CAD build for the part. Positions are in the model's coordinates, mm. Face numbers are marked on the shaded views. A direction names the side the tool comes from. Round coordinates to 2 decimals unless told otherwise and drop trailing zeros. Loops run counter-clockwise (first coordinate to the right, second up) from the corner with the lowest first, then second, coordinate; pieces in that order, holes last.
from build123d import *

# Parameters (mm, degrees)
SKETCH008_W     = 125
SKETCH008_H     = 60
PAD007_DEPTH    = 15
SKETCH009_W     = 115
SKETCH009_H     = 45
POCKET001_DEPTH = 10
SKETCH010_W     = 5
SKETCH010_H     = 45
PAD008_DEPTH    = 10
PAD009_DEPTH    = 15
PAD010_DEPTH    = 25
POCKET002_DEPTH = 122.392039
POCKET003_DEPTH = 62
PAD011_DEPTH    = 25
POCKET004_DEPTH = 22
FILLET006_R     = 1
FILLET007_R     = 1
FILLET008_R     = 1
FILLET009_R     = 1
FILLET010_R     = 2
PAD012_DEPTH    = 40
SKETCH019_W     = 26.11364
SKETCH019_H     = 14.637775
POCKET005_DEPTH = 11
POCKET006_DEPTH = 12
FILLET011_R     = 2
FILLET012_R     = 2


with BuildPart() as part:
    # Sketch008 → Pad007 (new body)
    with BuildSketch(Plane.XY):
        with Locations((97.753377, 76.478924)):
            Rectangle(SKETCH008_W, SKETCH008_H)
    extrude(amount=PAD007_DEPTH)

    # Sketch009 (on Face6 of Pad007) → Pocket001 (cut)
    with BuildSketch(Plane.XY.offset(15)):
        with Locations((97.753377, 73.978924)):
            Rectangle(SKETCH009_W, SKETCH009_H)
    extrude(amount=-POCKET001_DEPTH, mode=Mode.SUBTRACT)

    # Sketch010 (on Face11 of Pocket001) → Pad008 (join)
    with BuildSketch(Plane.XY.offset(5)):
        with Locations((97.753377, 73.978924)):
            Rectangle(SKETCH010_W, SKETCH010_H)
    extrude(amount=PAD008_DEPTH)

    # Sketch011 (on Face4 of Pad008) → Pad009 (join)
    with BuildSketch(Plane(origin=(0, 0, 0), x_dir=(1, 0, 0), z_dir=(0, 0, -1))):
        Polygon((40.253377, -103.478924), (155.253377, -103.478924), (142.543141, -146.646619), (97.753377, -168.869964), (52.963613, -146.646619), align=None)
    extrude(amount=-PAD009_DEPTH)

    # Sketch012 (on Face10 of Pad009) → Pad010 (join)
    with BuildSketch(Plane(origin=(0, 0, 0), x_dir=(1, 0, 0), z_dir=(0, 0, -1))):
        Polygon((35.753377, -91.478924), (35.753377, -61.478924), (36.388107, -46.478925), (9.764659, -46.478925), (-16.208147, -61.478924), (-16.208147, -91.478924), (9.764667, -106.478923), (35.753377, -106.478923), align=None)
    extrude(amount=-PAD010_DEPTH)

    # Sketch014 (on Face12 of Pad010) → Pocket002 (cut, through all)
    with BuildSketch(Plane.XZ.offset(-46.478925)):
        Polygon((21.625628, 4), (31.014697, 39.040485), (16.014696, 39.040485), (6.625628, 34.478157), (6.625628, 4), align=None)
    extrude(amount=-POCKET002_DEPTH, mode=Mode.SUBTRACT)

    # Sketch015 (on Face8 of Pocket002) → Pocket003 (cut)
    with BuildSketch(Plane.XZ.offset(-46.478925)):
        Polygon((2.97068, 27.121502), (-3.224708, 4), (-11.224708, 4), (-11.224708, 27.121502), align=None)
    extrude(amount=-POCKET003_DEPTH, mode=Mode.SUBTRACT)

    # Sketch016 (on Face2 of Pocket003) → Pad011 (join)
    with BuildSketch(Plane(origin=(0, 0, 0), x_dir=(1, 0, 0), z_dir=(0, 0, -1))):
        with BuildLine():
            ThreePointArc((160.253377, -106.478924), (190.253377, -76.478924), (160.253377, -46.478924))
            Line((160.253377, -46.478924), (158.253377, -46.478924))
            Line((158.253377, -46.478924), (158.253377, -106.478924))
            Line((158.253377, -106.478924), (160.253377, -106.478924))
        make_face()
    extrude(amount=-PAD011_DEPTH)

    # Sketch017 (on Face34 of Pad011) → Pocket004 (cut)
    with BuildSketch(Plane.XY.offset(25)):
        with BuildLine():
            ThreePointArc((160.253377, 49.478924), (187.253377, 76.478924), (160.253377, 103.478924))
            Line((160.253377, 103.478924), (160.253377, 49.478924))
        make_face()
    extrude(amount=-POCKET004_DEPTH, mode=Mode.SUBTRACT)

    # Fillet006
    fillet006_edges = [part.edges().sort_by_distance(p)[0] for p in [
        (158.253377, 76.478924, 25),
    ]]
    fillet(fillet006_edges, radius=FILLET006_R)

    # Fillet007
    fillet007_edges = [part.edges().sort_by_distance(p)[0] for p in [
        (31.502969, 106.478923, 25),
        (27.252561, 76.478924, 25),
        (31.820334, 46.478925, 25),
        (36.070742, 53.978925, 25),
        (35.753377, 83.978924, 25),
    ]]
    fillet(fillet007_edges, radius=FILLET007_R)

    # Fillet008
    fillet008_edges = [part.edges().sort_by_distance(p)[0] for p in [
        (2.402225, 76.478922, 25),
        (4.513926, 49.511365, 25),
        (6.625628, 76.478922, 25),
        (4.513926, 103.446479, 25),
    ]]
    fillet(fillet008_edges, radius=FILLET008_R)

    # Fillet009
    fillet009_edges = [part.edges().sort_by_distance(p)[0] for p in [
        (-16.208147, 76.478924, 25),
        (-13.716428, 60.039889, 25),
        (-11.224708, 76.478924, 25),
        (-13.716428, 92.917959, 25),
    ]]
    fillet(fillet009_edges, radius=FILLET009_R)

    # Fillet010
    fillet010_edges = [part.edges().sort_by_distance(p)[0] for p in [
        (127.753377, 51.478924, 15),
        (155.253377, 73.978924, 15),
        (100.253377, 73.978924, 15),
        (95.253377, 73.978924, 15),
        (67.753377, 51.478924, 15),
        (40.253377, 73.978924, 15),
    ]]
    fillet(fillet010_edges, radius=FILLET010_R)

    # Sketch018 (on DatumPlane) → Pad012 (join)
    with BuildSketch(Plane(origin=(138.35197, 76.478924, 12.5), x_dir=(0, 0, -1), z_dir=(1, 0, 0))):
        Polygon((0, 32.455163), (-41.423717, 43.554615), (0, 43.554615), align=None)
    extrude(amount=-PAD012_DEPTH)

    # Sketch019 (on Face25 of Pad012) → Pocket005 (cut)
    with BuildSketch(Plane(origin=(0, 120.033539, 0), x_dir=(-1, 0, 0), z_dir=(0, 1, 0))):
        with Locations((-120.645542, 22.318887)):
            Rectangle(SKETCH019_W, SKETCH019_H)
    extrude(amount=-POCKET005_DEPTH, mode=Mode.SUBTRACT)

    # Sketch020 (on Face47 of Pocket005) → Pocket006 (cut)
    with BuildSketch(Plane.XY.offset(15)):
        Polygon((50.450993, 122.512529), (145.055761, 122.512529), (138.543141, 144.6313), (97.753377, 164.869964), (56.963613, 144.6313), align=None)
    extrude(amount=-POCKET006_DEPTH, mode=Mode.SUBTRACT)

    # Fillet011
    fillet011_edges = [part.edges().sort_by_distance(p)[0] for p in [
        (53.707303, 133.571915, 15),
        (77.358495, 154.750632, 15),
        (118.148259, 154.750632, 15),
        (141.799451, 133.571915, 15),
    ]]
    fillet(fillet011_edges, radius=FILLET011_R)

    # Fillet012
    fillet012_edges = [part.edges().sort_by_distance(p)[0] for p in [
        (118.35197, 120.033539, 53.923717),
    ]]
    fillet(fillet012_edges, radius=FILLET012_R)


solid = part.part
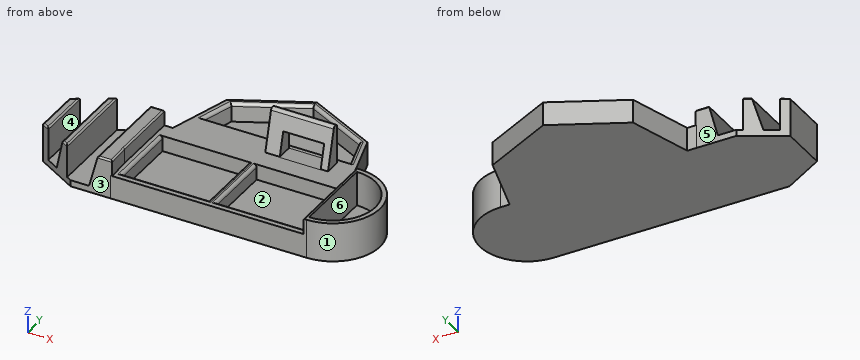
Item 1: Cut at C-C (z = 36). List the corners of the cut face in (x, y).
Verdict:
outline: (98.35, 115.23) - (138.35, 115.23) - (138.35, 120.03) - (98.35, 120.03) - close
Item 2: Flat gauge pins, fed straight in: P1, Ø4, axis at x = 72, z = 8.5, coming from the +Y side; P2, Ø4, axis at x = 75.5, y = 145.5, coming from the -Z side; P3, Ø1, axis at y = 93, z = 11.5, coming from the +X side; P4, Ø22, axis at y = 69.5, z = 17.5, coming from the +X side. Where does each tip first touch, or does it go through?
Verdict:
P1: stops at y = 157.08
P2: stops at z = 0
P3: stops at x = 185.62
P4: stops at x = 190.25
Item 3: Wall check: L1, parallel to Y at x = 120, z = 13; L2, parallel to X at y = 66.5, z = 9.5; L3, parallel to Y at x = 113, z = 7.5. Give the ranges that are in metal, low to high.
Verdict:
L1: y = 46.48 to 51.48, 96.48 to 122.51, 153.83 to 157.83
L2: x = -16.21 to -11.22, -1.75 to 6.63, 23.1 to 40.25, 95.25 to 100.25, 155.25 to 160.25, 185.34 to 188.55
L3: y = 46.48 to 51.48, 96.48 to 122.51, 157.31 to 161.31
Item 4: Cut at A-A (z = 21.5). List the corners of the cut face in (x, y).
Verdict:
outline: (-16.21, 61.48) - (-11.22, 58.6) - (-11.22, 94.36) - (-16.21, 91.48) - close; (1.46, 51.27) - (6.63, 48.29) - (6.63, 104.67) - (1.46, 101.69) - close; (26.31, 46.48) - (36.39, 46.48) - (35.75, 61.48) - (35.75, 106.48) - (26.31, 106.48) - close; (98.35, 111.35) - (107.59, 111.35) - (107.59, 120.03) - (98.35, 120.03) - close; (133.7, 111.35) - (138.35, 111.35) - (138.35, 120.03) - (133.7, 120.03) - close; (158.25, 46.48) - (160.25, 46.48) arc R30 ccw to (160.25, 106.48) - (158.25, 106.48) - close; hole (160.25, 49.48) arc R27 ccw to (160.25, 103.48) - close
Item 5: Cut at B-B (x = 12). List the corners of the cut face in (y, z), plus the area to 3 significant figures.
Verdict:
outline: (46.48, 0) - (106.48, 0) - (106.48, 4) - (46.48, 4) - close
area: 240 mm2
Item 6: Mould opens along Y. For the marked faces 1, 2 and 3 say: released by +Y, released by -Y, zero draft, split by the parting line, or undercut.
Verdict:
face 1: split by the parting line
face 2: undercut
face 3: released by -Y
Item 7: 3-axis set-ups, long thin cutter, end or side, ignore diameter. For the marked faces 4, 5 and 6: which of +Z, -Z, +X, -X, +Y, -Y reach the whole face in a straight line?
Verdict:
face 4: +Z, +Y, -Y
face 5: +Z, -Z, -X, +Y
face 6: +Z
